Autodesk Inventor part; units mm, degrees
ref_plane "YZ Plane" through (0, 0, 0) normal (1, 0, 0) x (0, 1, 0)
ref_plane "XZ Plane" through (0, 0, 0) normal (0, 1, 0) x (-1, 0, 0)
ref_plane "XY Plane" through (0, 0, 0) normal (0, 0, 1) x (1, 0, 0)
sketch "Sketch1" plane through (0, 0, 0) normal (0, 0, 1) x (1, 0, 0)
  line L0 (0, 2.8582) -> (0, -2.8582) construction
  line L1 (-5.7775, 0) -> (5.7775, 0) construction
  line L2 (-75, -70.5) -> (75, -70.5)
  line L3 (75, -70.5) -> (75, 70.5)
  line L4 (75, 70.5) -> (-75, 70.5)
  line L5 (-75, 70.5) -> (-75, -70.5)
  line L6 (-75, -70.5) -> (75, 70.5) construction
  line L7 (75, -70.5) -> (-75, 70.5) construction
  point P0 (0, 0)
  point P1 (0, 0)
  dimension "d0" = 150
  dimension "d1" = 141
extrude "Extrusion1" add sketch "Sketch1" along normal blind 5
sketch "Sketch2" plane through (0, 0, 5) normal (0, 0, 1) x (1, 0, 0)
  line L0 (-75, -70.5) -> (75, -70.5)
  line L1 (0, -70.5) -> (-15, -70.5)
  line L2 (-15, -70.5) -> (15, -70.5)
  line L3 (15, -70.5) -> (45, -70.5)
  line L4 (-15, -70.5) -> (-45, -70.5)
  line L5 (-15, -70.5) -> (15, -70.5)
  line L6 (15, -70.5) -> (15, -65.5)
  line L7 (15, -65.5) -> (-15, -65.5)
  line L8 (-15, -65.5) -> (-15, -70.5)
  line L9 (75, -70.5) -> (75, 70.5)
  line L10 (45, -70.5) -> (75, -70.5)
  line L11 (75, -70.5) -> (75, -65.5)
  line L12 (75, -65.5) -> (45, -65.5)
  line L13 (45, -65.5) -> (45, -70.5)
  line L14 (-75, 70.5) -> (-75, -70.5)
  line L15 (-45, -70.5) -> (-75, -70.5)
  line L16 (-75, -70.5) -> (-75, -65.5)
  line L17 (-75, -65.5) -> (-45, -65.5)
  line L18 (-45, -65.5) -> (-45, -70.5)
  line L19 (75, -70.5) -> (75, -55.5)
  line L20 (75, -55.5) -> (75, -25.5)
  line L21 (75, -25.5) -> (75, 4.5)
  line L22 (75, 4.5) -> (75, 34.5)
  line L23 (75, 34.5) -> (75, 64.5)
  line L24 (75, -25.5) -> (70, -25.5)
  line L25 (70, -25.5) -> (70, 6.5)
  line L26 (70, 6.5) -> (75, 6.5)
  line L27 (75, 6.5) -> (75, -25.5)
  line L28 (75, 70.5) -> (-75, 70.5)
  line L29 (75, 34.5) -> (70, 34.5)
  line L30 (70, 34.5) -> (70, 70.5)
  line L31 (70, 70.5) -> (75, 70.5)
  line L32 (75, 70.5) -> (75, 34.5)
  line L33 (-75, -25.5) -> (-70, -25.5)
  line L34 (-70, -25.5) -> (-70, 6.5)
  line L35 (-70, 6.5) -> (-75, 6.5)
  line L36 (-75, 6.5) -> (-75, -25.5)
  line L37 (-75, 34.5) -> (-70, 34.5)
  line L38 (-70, 34.5) -> (-70, 70.5)
  line L39 (-70, 70.5) -> (-75, 70.5)
  line L40 (-75, 70.5) -> (-75, 34.5)
  line L41 (0, 70.5) -> (-15, 70.5)
  line L42 (-15, 70.5) -> (15, 70.5)
  line L43 (15, 70.5) -> (45, 70.5)
  line L44 (-15, 70.5) -> (-45, 70.5)
  line L45 (-75, 70.5) -> (-45, 70.5)
  line L46 (-45, 70.5) -> (-45, 65.5)
  line L47 (-45, 65.5) -> (-75, 65.5)
  line L48 (-75, 65.5) -> (-75, 70.5)
  line L49 (-15, 70.5) -> (15, 70.5)
  line L50 (15, 70.5) -> (15, 65.5)
  line L51 (15, 65.5) -> (-15, 65.5)
  line L52 (-15, 65.5) -> (-15, 70.5)
  line L53 (45, 70.5) -> (75, 70.5)
  line L54 (75, 70.5) -> (75, 65.5)
  line L55 (75, 65.5) -> (45, 65.5)
  line L56 (45, 65.5) -> (45, 70.5)
  line L57 (-75, -25.5) -> (-67, -25.5)
  line L58 (-67, -25.5) -> (-67, -70.5)
  line L59 (-67, -70.5) -> (-75, -70.5)
  line L60 (-75, -70.5) -> (-75, -25.5)
  line L61 (-75, 6.5) -> (-70, 6.5)
  line L62 (-70, 6.5) -> (-70, 34.5)
  line L63 (-70, 34.5) -> (-75, 34.5)
  line L64 (-75, 34.5) -> (-75, 6.5)
  line L65 (70, 34.5) -> (75, 34.5)
  line L66 (75, 34.5) -> (75, 6.5)
  line L67 (75, 6.5) -> (70, 6.5)
  line L68 (70, 6.5) -> (70, 34.5)
  line L69 (70, -25.5) -> (75, -25.5)
  line L70 (75, -25.5) -> (75, -70.5)
  line L71 (75, -70.5) -> (70, -70.5)
  line L72 (70, -70.5) -> (70, -25.5)
  point P0 (0, 0)
  point P1 (-70, 70.5)
  point P2 (70, 65.5)
  point P3 (-70, 65.5)
  point P4 (70, 6.5)
  point P5 (-67, -65.5)
  point P6 (70, -65.5)
  dimension "d4" = 15
  dimension "d5" = 30
  dimension "d6" = 30
  dimension "d7" = 30
  dimension "d8" = 30
  dimension "d9" = 5
  dimension "d10" = 15
  dimension "d11" = 30
  dimension "d12" = 30
  dimension "d13" = 30
  dimension "d14" = 30
  dimension "d15" = 5
  dimension "d16" = 5
  dimension "d17" = 5
  dimension "d24" = 15
  dimension "d25" = 30
  dimension "d26" = 30
  dimension "d27" = 30
  dimension "d28" = 5
extrude "Extrusion2" cut sketch "Sketch2" against normal blind 8 contours L14 L17 L58 L0 | L58 L17 L18 L0 | L14 L33 L57 L58 L17 | L8 L7 L6 L0 | L14 L37 L62 L35 | L14 L28 L38 L47 | L13 L12 L72 L0 | L38 L28 L46 L47 | L72 L12 L9 L0 | L72 L24 L9 L12 | L28 L50 L51 L52 | L68 L29 L9 L26 | L55 L56 L28 L30 | L30 L28 L9 L55
sketch "Sketch3" plane through (0, 0, 5) normal (0, 0, 1) x (1, 0, 0)
  line L0 (-45, -45) -> (45, -45)
  line L1 (45, -45) -> (45, 45)
  line L2 (45, 45) -> (-45, 45)
  line L3 (-45, 45) -> (-45, -45)
  line L4 (-45, -45) -> (45, 45) construction
  line L5 (45, -45) -> (-45, 45) construction
  point P0 (0, 0)
  dimension "d20" = 90
  dimension "d21" = 90
extrude "Extrusion3" cut sketch "Sketch3" against normal blind 8
sketch "Sketch4" plane through (0, 0, 5) normal (0, 0, 1) x (1, 0, 0)
  line L0 (75, 34.5) -> (75, 65.5)
  line L1 (75, 65.5) -> (75, 21.5)
  line L2 (75, 21.5) -> (-125.9097, 21.5)
  line L3 (-125.9097, 21.5) -> (-125.9097, 76.2896)
  line L4 (-125.9097, 76.2896) -> (75, 76.2896)
  line L5 (75, 76.2896) -> (75, 21.5)
  point P0 (0, 0)
  dimension "d29" = 44
extrude "Extrusion4" cut sketch "Sketch4" against normal blind 15
properties part number "Plaat achter" material "S235"
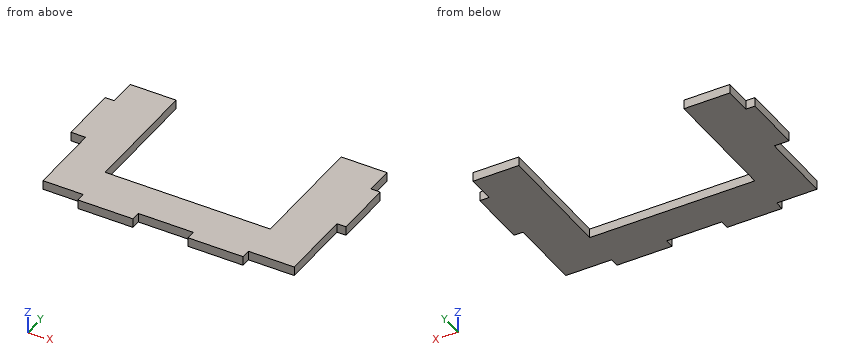
Read the model definition and answer for the solid it produces. Units are mm, in the model's axes. Round coordinates to 2 decimals unless told otherwise and drop trailing zeros. Write each loop counter-clockwise with the first axis right and the second up, starting at its lowest first coordinate (ties: lowest second). Pieces come first, ordered by that corner, then holes.
Q1. Find section A-A on y = -40. Determine the outline of the cut face in (x, z).
Values:
outline: (-67, 0) - (-45, 0) - (-45, 5) - (-67, 5) - close; (45, 0) - (70, 0) - (70, 5) - (45, 5) - close
Q2. Find section C-C on x = 52. Determine the outline of the cut face in (y, z).
Values:
outline: (-65.5, 0) - (21.5, 0) - (21.5, 5) - (-65.5, 5) - close
Q3. Find section B-B on z = 1.85. Determine the outline of the cut face in (x, y).
Values:
outline: (-75, -25.5) - (-67, -25.5) - (-67, -65.5) - (-45, -65.5) - (-45, -70.5) - (-15, -70.5) - (-15, -65.5) - (15, -65.5) - (15, -70.5) - (45, -70.5) - (45, -65.5) - (70, -65.5) - (70, -25.5) - (75, -25.5) - (75, 6.5) - (70, 6.5) - (70, 21.5) - (45, 21.5) - (45, -45) - (-45, -45) - (-45, 21.5) - (-70, 21.5) - (-70, 6.5) - (-75, 6.5) - close
Q4. Flat-ended cylindrical pins translate along their axes: P1, Ø2.5, axis at x = 55, z = 3.5, coming from the -Y side; P2, Ø2.5, axis at x = -72, z = 2, coming from the +Y side; P3, Ø2.5, axis at y = -69, z = 3.5, coming from the -X side. Find the tip coordinate at first contact, or state that the pin passes through.
Values:
P1: stops at y = -65.5
P2: stops at y = 6.5
P3: stops at x = -45
Q5. Straight lines are drawn through the part: line 1 (X direction, y = 7, z = 3); line 2 (X direction, y = -36.5, z = 2.65); line 3 (X direction, y = -61.5, z = 1.65). For each, find the intervals that lie inside material, in ascending order.
Values:
line 1: x = -70 to -45, 45 to 70
line 2: x = -67 to -45, 45 to 70
line 3: x = -67 to 70
Q6. Find section D-D on y = 4.5. Determine the outline of the cut face in (x, z).
Values:
outline: (-75, 0) - (-45, 0) - (-45, 5) - (-75, 5) - close; (45, 0) - (75, 0) - (75, 5) - (45, 5) - close
